For this review, take the finished solid that the model builds, in its own axes (mm). Face numbers are marked on the shaded views. Give positions to 0.01 mm unless a question says otherwise; leave off trailing zeros. Loops run counter-clockwise (first coordinate to the right, second up) from the corner with the lowest first, then second, coordinate; pieces in that order, holes last.
```python
from build123d import *

# Parameters (mm, degrees)
CIRPATTERN1_COUNT        = 3
CHAMFER1_SIZE            = 0.5
CHAMFER2_SIZE            = 1
CUT_EXTRUDE1_DEPTH       = 51.319429647
FILLET1_R                = 1.5
M3X0_5_TAPPED_HOLE1_D    = 2.5
CIRPATTERN2_COUNT        = 6
FILLET1_OF_CIRPATTERN2_R = 1.5
SKETCH10_W               = 1.207732619
SKETCH10_H               = 1.1
SKETCH11_W               = 3.151954219
SKETCH11_H               = 1.1
M3X0_5_TAPPED_HOLE2_D    = 2.5
CIRPATTERN3_COUNT        = 6
CHAMFER3_SIZE            = 0.5
CHAMFER4_SIZE            = 0.2


with BuildPart() as part:
    # Sketch2 → Revolve1 (revolve)
    with BuildSketch(Plane.XY, mode=Mode.PRIVATE) as revolve1_sk:
        Polygon((-4, 10), (-4, -6.5), (-3.1, -6.5), (-3.1, -9.5), (-4.1, -9.5), (-4.1, -7.5), (-6, -7.5), (-6, 10), (-7, 10), (-7, 17), (-32.65, 17), (-32.65, 20), (-5, 20), (-5, 11), align=None)
    revolve(revolve1_sk.sketch.rotate(Axis((0, 0, 0), (0, -1, 0)), 270), axis=Axis((0, 0, 0), (0, -1, 0)))

    # Sketch3 → Revolve2 (revolve)
    with BuildSketch(Plane.XY):
        Polygon((-22, 15), (-23, 15), (-23, 17), (-20.5, 17), (-20.5, 11), (-22, 11), align=None)
    revolve2 = revolve(axis=Axis((-20.5, 18.273035546, 0), (0, -1, 0)))

    # CirPattern1: Revolve2 ×3 about axis
    cirpattern1_axis = Axis((0, 0, 0), (0, 1, 0))
    for i in range(1, CIRPATTERN1_COUNT):
        add(revolve2.rotate(cirpattern1_axis, i * 360 / CIRPATTERN1_COUNT))

    # Chamfer1
    chamfer1_edges = [part.edges().sort_by_distance(p)[0] for p in [
        (0, 20, -32.65),
        (0, 17, -32.65),
    ]]
    chamfer(chamfer1_edges, length=CHAMFER1_SIZE)

    # Chamfer2
    chamfer2_edges = [part.edges().sort_by_distance(p)[0] for p in [
        (0, 20, -5),
    ]]
    chamfer(chamfer2_edges, length=CHAMFER2_SIZE)

    # Sketch6 → Cut-Extrude1 (cut, through all)
    with BuildSketch(Plane(origin=(0, 0, 0), x_dir=(1, 0, 0), z_dir=(0, 1, 0))):
        with BuildLine():
            Line((26.313380417, 4.222382152), (9.986832981, 4.611200171))
            ThreePointArc((9.986832981, 4.611200171), (9.526279442, 5.5), (8.986832981, 6.343250979))
            Line((8.986832981, 6.343250979), (16.813380417, 20.676864824))
            ThreePointArc((16.813380417, 20.676864824), (23.079577011, 13.325), (26.313380417, 4.222382152))
        make_face()
    cut_extrude1 = extrude(amount=CUT_EXTRUDE1_DEPTH, mode=Mode.SUBTRACT)

    # Fillet1
    fillet1_edges = [part.edges().sort_by_distance(p)[0] for p in [
        (26.313380417, 18.5, -4.222382152),
        (16.813380417, 18.5, -20.676864824),
        (8.986832981, 18.5, -6.343250979),
        (9.986832981, 18.5, -4.611200171),
    ]]
    fillet(fillet1_edges, radius=FILLET1_R)

    # M3x0.5 Tapped Hole1 (through all)
    with Locations(Plane(origin=(0, 20, 0), x_dir=(1, 0, 0), z_dir=(0, 1, 0))):
        with Locations((15, 0)):
            m3x0_5_tapped_hole1 = Hole(M3X0_5_TAPPED_HOLE1_D / 2)

    # CirPattern2: Cut-Extrude1, M3x0.5 Tapped Hole1 ×6 about axis
    cirpattern2_axis = Axis((0, 0, 0), (0, 1, 0))
    add([cut_extrude1.rotate(cirpattern2_axis, i * 360 / CIRPATTERN2_COUNT) for i in range(1, CIRPATTERN2_COUNT)], mode=Mode.SUBTRACT)
    add([m3x0_5_tapped_hole1.rotate(cirpattern2_axis, i * 360 / CIRPATTERN2_COUNT) for i in range(1, CIRPATTERN2_COUNT)], mode=Mode.SUBTRACT)

    # Fillet1 of CirPattern2
    fillet1_of_cirpattern2_edges = [part.edges().sort_by_distance(p)[0] for p in [
        (9.5, 18.5, -24.899246977),
        (-9.5, 18.5, -24.899246977),
        (-1, 18.5, -10.95445115),
        (1, 18.5, -10.95445115),
        (-16.813380417, 18.5, -20.676864824),
        (-26.313380417, 18.5, -4.222382152),
        (-9.986832981, 18.5, -4.611200171),
        (-8.986832981, 18.5, -6.343250979),
        (-26.313380417, 18.5, 4.222382152),
        (-16.813380417, 18.5, 20.676864824),
        (-8.986832981, 18.5, 6.343250979),
        (-9.986832981, 18.5, 4.611200171),
        (-9.5, 18.5, 24.899246977),
        (9.5, 18.5, 24.899246977),
        (1, 18.5, 10.95445115),
        (-1, 18.5, 10.95445115),
        (16.813380417, 18.5, 20.676864824),
        (26.313380417, 18.5, 4.222382152),
        (9.986832981, 18.5, 4.611200171),
        (8.986832981, 18.5, 6.343250979),
    ]]
    fillet(fillet1_of_cirpattern2_edges, radius=FILLET1_OF_CIRPATTERN2_R)

    # Sketch9 → Cut-Revolve1 (revolve, cut)
    with BuildSketch(Plane.XY, mode=Mode.PRIVATE) as cut_revolve1_sk:
        Polygon((-8.538708616, -5.4), (-5.75, -5.4), (-5.75, -6.5), (-6.5, -6.5), (-5.5, -7.5), (-8.538708616, -7.5), align=None)
    revolve(cut_revolve1_sk.sketch.rotate(Axis((0, 0, 0), (0, -1, 0)), 270), axis=Axis((0, 0, 0), (0, -1, 0)), mode=Mode.SUBTRACT)

    # Sketch10 → Cut-Revolve2 (revolve, cut)
    with BuildSketch(Plane.XY, mode=Mode.PRIVATE) as cut_revolve2_sk:
        with Locations((-6.35386631, 5.45)):
            Rectangle(SKETCH10_W, SKETCH10_H)
    revolve(cut_revolve2_sk.sketch.rotate(Axis((0, 0, 0), (0, 1, 0)), 90), axis=Axis((0, 0, 0), (0, 1, 0)), mode=Mode.SUBTRACT)

    # Sketch11 → Cut-Revolve3 (revolve, cut)
    with BuildSketch(Plane.XY, mode=Mode.PRIVATE) as cut_revolve3_sk:
        with Locations((-7.32597711, 3.15)):
            Rectangle(SKETCH11_W, SKETCH11_H)
    revolve(cut_revolve3_sk.sketch.rotate(Axis((0, 0, 0), (0, -1, 0)), 270), axis=Axis((0, 0, 0), (0, -1, 0)), mode=Mode.SUBTRACT)

    # M3x0.5 Tapped Hole2 (through all)
    with Locations(Plane(origin=(0, 20, 0), x_dir=(1, 0, 0), z_dir=(0, 1, 0))):
        with Locations((0, 30)):
            m3x0_5_tapped_hole2 = Hole(M3X0_5_TAPPED_HOLE2_D / 2)

    # CirPattern3: M3x0.5 Tapped Hole2 ×6 about axis
    cirpattern3_axis = Axis((0, 0, 0), (0, 1, 0))
    for i in range(1, CIRPATTERN3_COUNT):
        add(m3x0_5_tapped_hole2.rotate(cirpattern3_axis, i * 360 / CIRPATTERN3_COUNT), mode=Mode.SUBTRACT)

    # Chamfer3
    chamfer3_edges = [part.edges().sort_by_distance(p)[0] for p in [
        (4.996137366, 20, -17.51037111),
        (0, 20, -26.65),
        (0, 20, -11),
        (-4.996137366, 20, -17.51037111),
        (8.646973206, 20, -24.619750438),
        (0.909363746, 20, -11.185375999),
        (-0.909363746, 20, -11.185375999),
        (-8.646973206, 20, -24.619750438),
        (-12.666357528, 20, -13.081967435),
        (-23.079577011, 20, -13.325),
        (-9.526279442, 20, -5.5),
        (-17.662494894, 20, -4.428403676),
        (-16.997842711, 20, -19.798373681),
        (-9.232137893, 20, -6.380220105),
        (-10.141501639, 20, -4.805155894),
        (-25.644815917, 20, -4.821376756),
        (-17.662494894, 20, 4.428403676),
        (-23.079577011, 20, 13.325),
        (-9.526279442, 20, 5.5),
        (-12.666357528, 20, 13.081967435),
        (-25.644815917, 20, 4.821376756),
        (-10.141501639, 20, 4.805155894),
        (-9.232137893, 20, 6.380220105),
        (-16.997842711, 20, 19.798373681),
        (-4.996137366, 20, 17.51037111),
        (0, 20, 26.65),
        (0, 20, 11),
        (4.996137366, 20, 17.51037111),
        (-8.646973206, 20, 24.619750438),
        (-0.909363746, 20, 11.185375999),
        (0.909363746, 20, 11.185375999),
        (8.646973206, 20, 24.619750438),
        (12.666357528, 20, 13.081967435),
        (23.079577011, 20, 13.325),
        (9.526279442, 20, 5.5),
        (17.662494894, 20, 4.428403676),
        (16.997842711, 20, 19.798373681),
        (9.232137893, 20, 6.380220105),
        (10.141501639, 20, 4.805155894),
        (25.644815917, 20, 4.821376756),
        (17.662494894, 20, -4.428403676),
        (23.079577011, 20, -13.325),
        (9.526279442, 20, -5.5),
        (12.666357528, 20, -13.081967435),
        (25.644815917, 20, -4.821376756),
        (10.141501639, 20, -4.805155894),
        (9.232137893, 20, -6.380220105),
        (16.997842711, 20, -19.798373681),
    ]]
    chamfer(chamfer3_edges, length=CHAMFER3_SIZE)

    # Chamfer4
    chamfer4_edges = [part.edges().sort_by_distance(p)[0] for p in [
        (-19, 11, 0),
        (9.5, 11, 16.454482672),
        (9.5, 11, -16.454482672),
    ]]
    chamfer(chamfer4_edges, length=CHAMFER4_SIZE)


solid = part.part
```
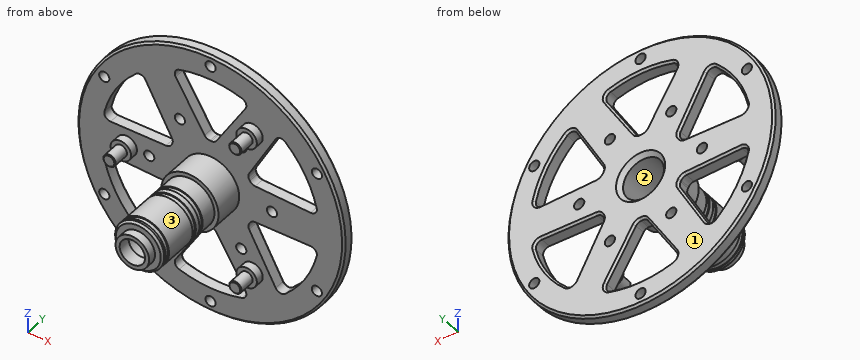
Item 1: For L1, parallel to X at y = 12.5, z = 0; L2, parallel to X at y = -8.1, z = 0; L3, parallel to Y at x = -10, z = -15, list the stretches that pass through material, from the lowest coordinate up.
Answer:
L1: x = -22 to -19, -7 to -5, 5 to 7
L2: x = -4.1 to -3.1, 3.1 to 4.1
L3: y = 17 to 20
Item 2: Take a section at B-B on z = 0. State how many separate pieces and enclosed holes the cut face has, and give its area (3 significant figures).
Answer:
separate pieces: 4
enclosed holes: 0
area: 274 mm2
Item 3: Take a section at A-A on y = -1.75. Give the boundary of the cut face in (x, z), and give its area (3 significant figures).
Answer:
outline: circle Ø12 at (0, 0); hole circle Ø8 at (0, 0)
area: 62.8 mm2
Item 4: Clearance check with flat-ended pins moving along their axes: pin 1 Ø5.5 at (x, z) = (10, -16.5) entering from -Y; pin 2 Ø3 at (x, y) = (5, -6) entering from +Z; pin 3 Ø5 at (x, z) = (-0.5, 12) entering from -Y. State where each tip first meets the part, or that it passes through.
Answer:
pin 1: stops at y = 11
pin 2: stops at z = 4.81
pin 3: stops at y = 17
Item 5: The part is to be moulded in two halves that separate along X. For the marked faces 1, 2 and 3, say which applies: released by +X, released by -X, zero draft, split by the parting line, or undercut.
Answer:
face 1: zero draft
face 2: undercut
face 3: split by the parting line
